Source: CAD feature listing. Evaluate the final solid. Frame: model axes, mm. A direction names the side the tool comes from. Give positions to 0.01 mm unless a question says otherwise; leave off trailing zeros. Order: outer loops, then holes, each group sorted by start corner. A loop starts at its lowest first (then second) coordinate and runs counter-clockwise, first axis right, second up.
from build123d import *

# Parameters (mm, degrees)
CROQUIS1_W              = 49.8
CROQUIS1_H              = 39.8
CROQUIS1_R              = 2.7
SALIENTE_EXTRUIR1_DEPTH = 1.2
REDONDEO1_R             = 3
CROQUIS2_W              = 6
CROQUIS2_H              = 7
SALIENTE_EXTRUIR2_DEPTH = 7


with BuildPart() as part:
    # Croquis1 → Saliente-Extruir1 (new body)
    with BuildSketch(Plane.XY):
        with Locations((-31.963412372, -3.757931034)):
            Rectangle(CROQUIS1_W, CROQUIS1_H)
        with Locations((-52.963412372, 12.342068966)):
            Circle(CROQUIS1_R, mode=Mode.SUBTRACT)
        with Locations((-10.963412372, 12.342068966)):
            Circle(CROQUIS1_R, mode=Mode.SUBTRACT)
        with Locations((-10.963412372, -19.657931034)):
            Circle(CROQUIS1_R, mode=Mode.SUBTRACT)
        with Locations((-52.963412372, -19.657931034)):
            Circle(CROQUIS1_R, mode=Mode.SUBTRACT)
    extrude(amount=SALIENTE_EXTRUIR1_DEPTH)

    # Redondeo1
    redondeo1_edges = [part.edges().sort_by_distance(p)[0] for p in [
        (-56.863412372, 16.142068966, 0.6),
        (-7.063412372, 16.142068966, 0.6),
        (-7.063412372, -23.657931034, 0.6),
        (-56.863412372, -23.657931034, 0.6),
    ]]
    fillet(redondeo1_edges, radius=REDONDEO1_R)

    # Croquis2 → Saliente-Extruir2 (add)
    with BuildSketch(Plane.XY.offset(1.2)):
        with Locations((-43.595564528, 12.642068966)):
            Rectangle(CROQUIS2_W, CROQUIS2_H)
    extrude(amount=SALIENTE_EXTRUIR2_DEPTH)


solid = part.part
1) Section query C-C on y = -1. Output: boundary loops of the cut face in (x, z).
Checks:
outline: (-56.86, 0) - (-7.06, 0) - (-7.06, 1.2) - (-56.86, 1.2) - close
2) Reachability of faces 4 (the face through (-44, 9.142, 5)), 5 (the face through (-9.512, 14.619, 0.592)), 6 (the face through (-46.596, 13, 5)) from +Z, -Z, +X, -X, +Y, -Y: full face, straight path, thin tool, end or side. Return the list, or none.
Checks:
face 4: +Z, +X, -X, -Y
face 5: +Z, -Z
face 6: +Z, -X, +Y, -Y
3) Pull-direction query (Y, two-part tool) for faces 1 (the face through (-50.388, 13.153, 0.592)), 2 (the face through (-40.596, 13, 5)), 3 (the face through (-7.97, 15.29, 0.61)); classes: +Y half, -Y half, draft (parallel to the pull), parting line (faces both ways), or undercut.
Checks:
face 1: undercut
face 2: draft
face 3: +Y half
4) First-contact query: pin 1 Ø1.8 at (x, z) = (-45, 4.5) entering from -Y; pin 2 Ø3.5 at (y, z) = (14, 6) entering from -X; pin 3 Ø7 at (x, y) = (-52.96, -19.66) entering from +Z. Flat tips, straight axial feed; report the tip coordinate or a pass-through.
Checks:
pin 1: stops at y = 9.14
pin 2: stops at x = -46.6
pin 3: stops at z = 1.2
5) Section query A-A on y = 14. Output: boundary loops of the cut face in (x, z).
Checks:
outline: (-56.74, 0) - (-55.09, 0) - (-55.09, 1.2) - (-56.74, 1.2) - close; (-50.83, 0) - (-13.09, 0) - (-13.09, 1.2) - (-40.6, 1.2) - (-40.6, 8.2) - (-46.6, 8.2) - (-46.6, 1.2) - (-50.83, 1.2) - close; (-8.83, 0) - (-7.19, 0) - (-7.19, 1.2) - (-8.83, 1.2) - close
6) Ray query, L1, parallel to Z at x = -10.5, y = -16; L2, parallel to Y at x = -45, z = 4.75; L3, parallel to X at y = 10.5, z = 3.5. Return the intervals inside material, ascending.
Checks:
L1: z = 0 to 1.2
L2: y = 9.14 to 16.14
L3: x = -46.6 to -40.6
7) Section query B-B on x = -20.5. Output: boundary loops of the cut face in (y, z).
Checks:
outline: (-23.66, 0) - (16.14, 0) - (16.14, 1.2) - (-23.66, 1.2) - close
